Here's how the part is built. I have some questions about the finished solid (model axes, mm). Face numbers are marked on the shaded views. A direction names the side the tool comes from. Coordinates: 2 decimals unless noted, no trailing zeros. Write each loop counter-clockwise with the first axis right and the second up, starting at its lowest first coordinate (ties: lowest second). Pieces come first, ordered by that corner, then holes. Notation, with made-up numbers: M -27.75,-18 L -7.75,-18 A13 ccw -7.75,2 Z; hole C 15.25,16 d2. An arc over 180 degrees is marked long. Use one line per item in the form item = value. Start each with the question number.
1. I want a section at A-A, the plane x = 12.7. List the corners of the cut face in (y, z) for me.
2. I want a section at D-D, the plane x = -13. List the corners of the cut face in (y, z) for me.
3. I want a section at B-B, the plane y = 2. Count the separate pieces of the cut face and the enclosed holes in it, plus the area to 3 significant figures.
4. Please list where these lines run through material, in increasing order: line 1 along Z through (x, y) = (12.7, 4.5); line 2 along X through (y, z) = (1.75, -12.7); line 3 along X through (y, z) = (0.5, -11). Write a range as [from, to].
5. On a 3-axis mill with a long thin cutter (end or side, diameter ignored), from which of +Z, -Z, +X, -X, +Y, -Y can I reach the whole of each face in a straight line? I mean the marked faces 1, 2, 3, 4 and 5. Say none if no direction works.
6. I'm going to push flat-ended pins straight in: pin 1 Ø3.5 at (x, z) = (12.7, 12.7) entering from -Y; pin 2 Ø9 at (x, z) = (-12.7, 12.7) entering from -Y; pin 3 Ø1.9 at (x, y) = (23.5, 2.5) entering from -Z; pin 4 Ø2.5 at (y, z) = (2.5, -32) entering from +X. Where does each tip first touch, or does it pass through?
7. Thinking about a two-plate mould opening in X: for the marked faces 6, 7, 8 and 9, which applies, released by +X, released by -X, zero draft, split by the parting line, or undercut?
8. I want a section at C-C, the plane z = 12.7. List the corners of the cut face in (x, y) for me, plus the area to 3 significant figures.
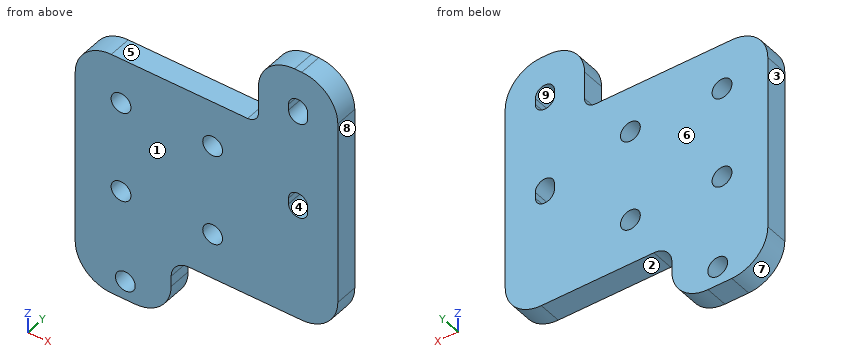
from build123d import *

# Parameters (mm, degrees)
BOSS_EXTRUDE1_DEPTH  = 6.35
M5_CLEARANCE_HOLE1_D = 5.5
CUT_EXTRUDE2_DEPTH   = 7.35
FILLET1_R            = 10
FILLET2_R            = 3
FILLET3_R            = 5


with BuildPart() as part:
    # Sketch1 → Boss-Extrude1 (new body)
    with BuildSketch(Plane(origin=(0, 0, 0), x_dir=(1, 0, 0), z_dir=(0, 1, 0))):
        Polygon((25.4, -25.4), (-25.4, -25.4), (-25.4, 25.4), (-25.4, 43.35), (1.2, 43.35), (1.2, 25.4), (25.4, 25.4), (47.4, 25.4), (47.4, -46.04), (36.4, -46.04), (25.4, -46.04), align=None)
    extrude(amount=BOSS_EXTRUDE1_DEPTH)

    # M5 Clearance Hole1 (through all)
    with Locations(Plane(origin=(0, 6.35, 0), x_dir=(1, 0, 0), z_dir=(0, 1, 0))):
        with Locations((-12.7, 12.7), (12.7, 12.7), (12.7, -12.7), (-12.7, -12.7), (-11.5, 38.1)):
            Hole(M5_CLEARANCE_HOLE1_D / 2)

    # Sketch7 → Cut-Extrude2 (cut, through all)
    with BuildSketch(Plane(origin=(0, 6.35, 0), x_dir=(1, 0, 0), z_dir=(0, 1, 0))):
        with BuildLine():
            Line((33.75, -33.4), (33.75, -35.04))
            ThreePointArc((33.75, -35.04), (36.4, -37.69), (39.05, -35.04))
            Line((39.05, -35.04), (39.05, -33.4))
            ThreePointArc((39.05, -33.4), (36.4, -30.75), (33.75, -33.4))
        make_face()
        with BuildLine():
            Line((33.75, -6.36), (33.75, -8))
            ThreePointArc((33.75, -8), (36.4, -10.65), (39.05, -8))
            Line((39.05, -8), (39.05, -6.36))
            ThreePointArc((39.05, -6.36), (36.4, -3.71), (33.75, -6.36))
        make_face()
    extrude(amount=-CUT_EXTRUDE2_DEPTH, mode=Mode.SUBTRACT)

    # Fillet1
    fillet1_edges = [part.edges().sort_by_distance(p)[0] for p in [
        (-25.4, 3.175, -43.35),
        (1.2, 3.175, -43.35),
        (47.4, 3.175, -25.4),
        (47.4, 3.175, 46.04),
        (25.4, 3.175, 46.04),
        (-25.4, 3.175, 25.4),
    ]]
    fillet(fillet1_edges, radius=FILLET1_R)

    # Fillet2
    fillet2_edges = [part.edges().sort_by_distance(p)[0] for p in [
        (25.4, 3.175, 25.4),
    ]]
    fillet(fillet2_edges, radius=FILLET2_R)

    # Fillet3
    fillet3_edges = [part.edges().sort_by_distance(p)[0] for p in [
        (1.2, 3.175, -25.4),
    ]]
    fillet(fillet3_edges, radius=FILLET3_R)


solid = part.part
Answer list:
q1.outline = M 0,-25.4 L 6.35,-25.4 L 6.35,-15.45 L 0,-15.45 Z; M 0,-9.95 L 6.35,-9.95 L 6.35,9.95 L 0,9.95 Z; M 0,15.45 L 6.35,15.45 L 6.35,25.4 L 0,25.4 Z
q2.outline = M 0,-43.35 L 6.35,-43.35 L 6.35,-40.4 L 0,-40.4 Z; M 0,-35.8 L 6.35,-35.8 L 6.35,-15.43 L 0,-15.43 Z; M 0,-9.97 L 6.35,-9.97 L 6.35,9.97 L 0,9.97 Z; M 0,15.43 L 6.35,15.43 L 6.35,25.4 L 0,25.4 Z
q3.separate_pieces = 1
q3.enclosed_holes = 7
q3.area = 4,330 mm²
q4.line_1 = [-25.4, -15.45], [-9.95, 9.95], [15.45, 25.4]
q4.line_2 = [-25.4, -15.45], [-9.95, 9.95], [15.45, 47.4]
q4.line_3 = [-25.4, -14.86], [-10.54, 10.54], [14.86, 47.4]
q5.face_1 = +Z, -Z, +X, -X, -Y
q5.face_2 = -Z, +X, +Y, -Y
q5.face_3 = +Z, -Z, -X, +Y, -Y
q5.face_4 = +Y, -Y
q5.face_5 = +Z, -X, +Y, -Y
q6.pin_1 = through
q6.pin_2 = 0
q6.pin_3 = -25.4
q6.pin_4 = 1.2
q7.face_6 = zero draft
q7.face_7 = released by -X
q7.face_8 = released by +X
q7.face_9 = undercut
q8.outline = M -25.4,0 L -15.45,0 L -15.45,6.35 L -25.4,6.35 Z; M -9.95,0 L 9.95,0 L 9.95,6.35 L -9.95,6.35 Z; M 15.45,0 L 47.4,0 L 47.4,6.35 L 15.45,6.35 Z
q8.area = 392 mm²
